Design review of the part built by this model. Coordinates are the model's own, in mm. Face numbers are marked on the shaded views. A direction names the side the tool comes from. Coordinates: 2 decimals unless noted, no trailing zeros. Order: outer loops, then holes, each group sorted by start corner. A loop starts at its lowest first (then second) coordinate and runs counter-clockwise, first axis right, second up. Notation, with made-up numbers: (-18, 10) -> (-6, 10) arc R21 cw to (-6, 14) -> close; hole circle Ø3 at (9.25, 71). An arc over 180 degrees is marked (long way). Use a Markdown table: item, result. Add a question column.
Q1. Add section D-D (y = -23). State the section outline as (x, z) points.
Q2. Add section B-B (z = 34). State the section outline as (x, y) points, then the cut area to 3 significant figures.
Q3. Insertion check: pin 1 (6 mm diameter, centred on x = -40.5, z = 28.5, fed in from -Y); pin 2 (3 mm diameter, centred on x = -110, z = 7, fed in from +Y); pin 3 (4 mm diameter, centred on x = -26, y = 22, fed in from +Z). Each pin has a flat end and moves straight along its axis. Give the tip position at first contact, or say it passes through.
Q4. Add section C-C (x = -21). State the section outline as (y, z) points, then the cut area to 3 significant figures.
Q5. Machinability: for the marked faces 1 and 2, which of the approach directions +Z, -Z, +X, -X, +Y, -Y give a long, thin tool a straight path to every point of the face, cutting with its end or side? Answer none if there is none.
Q6. Add section A-A (y = -13.5). State the section outline as (x, z) points, then the cut area to 3 significant figures.
Q7. Wall thickness on probe 1 along X at (y, z) = (-4, 15); probe 2 along Z at (x, y) = (-19.5, 1.5); probe 3 along Z at (x, y) = (-129.5, 25): over which ranges is each line inside the solid? List them lowest first.
Q8. The part is to be moulded in two halves that separate along X. For the marked faces 3, 4 and 5, say which applies: pulls with the +X half, pulls with the -X half, needs draft (parallel to the pull), parting line crosses it, or undercut.
from build123d import *

# Parameters (mm, degrees)
F1_DEPTH = 152.4
F2_W     = 12.700002
F2_H     = 38.1
F3_DEPTH = 38.101


with BuildPart() as f1:
    # F0 (on Right) → F1 (new body)
    with BuildSketch(Plane.YZ):
        with BuildLine():
            Line((-38.1, 0), (38.1, 0))
            ThreePointArc((38.1, 0), (0, 38.1), (-38.1, 0))
        make_face()
    extrude(amount=-F1_DEPTH)

    # F2 (on face) → F3 (cut, through all)
    with BuildSketch(Plane(origin=(0, 0, 0), x_dir=(1, 0, 0), z_dir=(0, 0, -1))):
        with Locations((-76.199999, 19.05)):
            Rectangle(F2_W, F2_H)
    extrude(amount=-F3_DEPTH, mode=Mode.SUBTRACT)


solid = f1.part
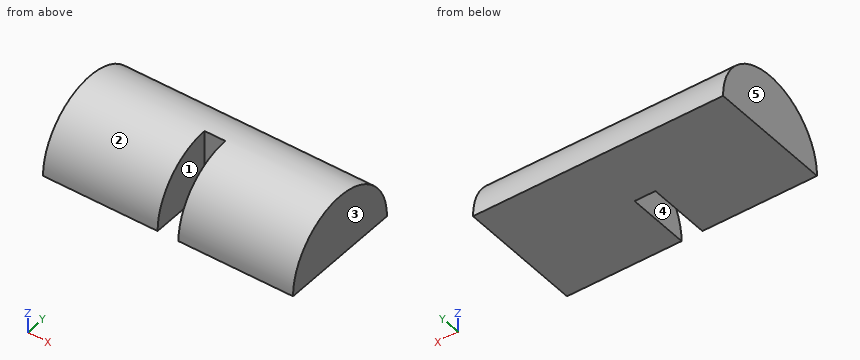
Established:
| question | item | result |
|---|---|---|
| 1 | outline | (-152.4, 0) -> (-82.55, 0) -> (-82.55, 30.37) -> (-152.4, 30.37) -> close; (-69.85, 0) -> (0, 0) -> (0, 30.37) -> (-69.85, 30.37) -> close |
| 2 | outline | (-152.4, -17.19) -> (-82.55, -17.19) -> (-82.55, 0) -> (-69.85, 0) -> (-69.85, -17.19) -> (0, -17.19) -> (0, 17.19) -> (-152.4, 17.19) -> close |
| 2 | area | 5,020 mm^2 |
| 3 | pin 1 | y = -28.31 |
| 3 | pin 2 | y = 37.7 |
| 3 | pin 3 | z = 32.43 |
| 4 | outline | (-38.1, 0) -> (38.1, 0) arc R38.1 ccw to start |
| 4 | area | 2,280 mm^2 |
| 5 | face 1 | +Z, -Z, -Y |
| 5 | face 2 | +Z, +X, -X |
| 6 | outline | (-152.4, 0) -> (-82.55, 0) -> (-82.55, 35.63) -> (-152.4, 35.63) -> close; (-69.85, 0) -> (0, 0) -> (0, 35.63) -> (-69.85, 35.63) -> close |
| 6 | area | 4,980 mm^2 |
| 7 | probe 1 | -152.4 to -82.55, -69.85 to 0 |
| 7 | probe 2 | 0 to 38.07 |
| 7 | probe 3 | 0 to 28.75 |
| 8 | face 3 | pulls with the +X half |
| 8 | face 4 | undercut |
| 8 | face 5 | pulls with the -X half |
